Could you check a few things on this model? Use its own coordinates, in mm. A direction names the side the tool comes from. Coordinates: 2 decimals unless noted, no trailing zeros. Loops run counter-clockwise (first coordinate to the right, second up) from the corner with the lowest first, then second, coordinate; pieces in that order, holes last. Notation, with made-up numbers: (-27.5, -36) -> (3.5, -36) arc R34 ccw to (3.5, -3) -> close; hole circle Ø1 at (-4, -20.75). An arc over 180 degrees is marked (long way). One line per question, with ' | ' between items.
Autodesk Inventor part; units mm, degrees
ref_plane "YZ Plane" through (0, 0, 0) normal (1, 0, 0) x (0, 1, 0)
ref_plane "XZ Plane" through (0, 0, 0) normal (0, 1, 0) x (-1, 0, 0)
sketch "スケッチ2" plane through (0, 0, 0) normal (0, 0, 1) x (1, 0, 0)
  circle A0 centre (0, 0) radius 15
  dimension "d2" = 30
extrude "押し出し1" add sketch "スケッチ2" against normal blind 60
sketch "スケッチ3" plane through (0, 0, -60) normal (0, 0, -1) x (-1, 0, 0)
  line L0 (37.5, 15) -> (-37.5, 15)
  line L1 (-37.5, 15) -> (-37.5, -15)
  line L2 (-37.5, -15) -> (37.5, -15)
  line L3 (37.5, -15) -> (37.5, 15)
  point P0 (0, 0)
  point P1 (0, 15)
  point P2 (37.5, 0)
  dimension "d5" = 30
  dimension "d6" = 75
extrude "押し出し2" add sketch "スケッチ3" along normal blind 100
sketch "スケッチ4" plane through (0, 0, 0) normal (0, 1, 0) x (-1, 0, 0)
  line L0 (63.5061, 71.4951) -> (-75.4219, 71.4951)
  line L1 (-75.4219, 71.4951) -> (-75.4219, -50)
  line L2 (-75.4219, -50) -> (63.5061, -50)
  line L3 (63.5061, -50) -> (63.5061, 71.4951)
  line L4 (-103.2075, 0) -> (91.2917, 0)
  point P0 (0, 0)
  dimension "d9" = 50
extrude "押し出し3" cut sketch "スケッチ4" against normal mid plane 100
properties part number "HandY"
1) If we section it at C-C on x = -23: Please give me the cut outline in (y, z), and give its area (3 significant figures).
Data:
outline: (-15, -160) -> (15, -160) -> (15, -60) -> (-15, -60) -> close | area: 3,000 mm²
2) I need wall thicknesses on line 1 along Z through (x, y) = (33, 9.5); line 2 along Y through (x, z) = (1, -57.5). Which ranges of each line are inside material? Lowest first, please. Write a range as from..to.
Data:
line 1: -160..-60 | line 2: -14.97..14.97
3) If we section it at B-B on x = -12.5: Please give me the cut outline in (y, z), and give its area (3 significant figures).
Data:
outline: (-15, -160) -> (15, -160) -> (15, -60) -> (8.29, -60) -> (8.29, -50) -> (-8.29, -50) -> (-8.29, -60) -> (-15, -60) -> close | area: 3,170 mm²
4) If we section it at A-A on y = 12: Please give me the cut outline in (x, z).
Data:
outline: (-37.5, -160) -> (37.5, -160) -> (37.5, -60) -> (9, -60) -> (9, -50) -> (-9, -50) -> (-9, -60) -> (-37.5, -60) -> close
5) We'd pull the mould along Z, two halves only. Please class faces 3 (the face through (37.5, 0, -109)), 4 (the face through (1, 0, -160)), 5 (the face through (-27, 0, -60)): pulls with the +Z half, pulls with the -Z half, needs draft (parallel to the pull), parting line crosses it, or undercut.
Data:
face 3: needs draft | face 4: pulls with the -Z half | face 5: pulls with the +Z half
6) On a 3-axis mill with a long thin cutter (end or side, diameter ignored), from which of +Z, -Z, +X, -X, +Y, -Y can I reach the whole of each face in a straight line? I mean faces 1 (the face through (-14.985, 0.66, -54.93)), 2 (the face through (0, 0, -50)). Say none if no direction works.
Data:
face 1: +Z | face 2: +Z, +X, -X, +Y, -Y
